Verification items for the finished model (mm, model axes). Face numbers are marked on the shaded views. A direction names the side the tool comes from. Coordinates: 2 decimals unless noted, no trailing zeros. Write each loop counter-clockwise with the first axis right and the second up, starting at its lowest first coordinate (ties: lowest second). Pieces come first, ordered by that corner, then holes. Notation, with made-up numbers: M 77,26.5 L 120,26.5 A21 cw 120,54.5 Z; hole C 52.5,33.25 d6. An arc over 180 degrees is marked long. Answer in a Markdown table with one row per item.
from build123d import *

# Parameters (mm, degrees)
F0_R     = 3
F0_R_2   = 1.5
F1_DEPTH = 2
F0_W     = 43.5258374241
F0_H     = 104
F2_DEPTH = 5
F4_R     = 6.5
F5_DEPTH = 4
F6_R     = 5
F7_R     = 8


# Not quite as in the source:
# - a feature names something its author has since deleted; it is built from what else it names


with BuildPart() as f1:
    # F0 (on Top) → F1 (new body)
    with BuildSketch(Plane.XY):
        Polygon((21, 52), (20, 52), (-20, 52), (-21, 52), (-21, -52), (-20, -52), (20, -52), (21, -52), align=None)
        with Locations((-13, -44)):
            Circle(F0_R, mode=Mode.SUBTRACT)
        with Locations((13, -44)):
            Circle(F0_R, mode=Mode.SUBTRACT)
        with Locations((-13, -8)):
            Circle(F0_R, mode=Mode.SUBTRACT)
        Polygon((-5, -16), (-5, -5), (5, -5), (5, -16), (16, -16), (16, -36), (5, -36), (5, -47), (-5, -47), (-5, -36), (-16, -36), (-16, -16), align=None, mode=Mode.SUBTRACT)
        with Locations((13, -8)):
            Circle(F0_R, mode=Mode.SUBTRACT)
        with Locations((-13, 8)):
            Circle(F0_R, mode=Mode.SUBTRACT)
        with Locations((13, 8)):
            Circle(F0_R, mode=Mode.SUBTRACT)
        with Locations((-13, 44)):
            Circle(F0_R, mode=Mode.SUBTRACT)
        Polygon((-5, 36), (-5, 47), (5, 47), (5, 36), (16, 36), (16, 16), (5, 16), (5, 5), (-5, 5), (-5, 16), (-16, 16), (-16, 36), align=None, mode=Mode.SUBTRACT)
        with Locations((13, 44)):
            Circle(F0_R, mode=Mode.SUBTRACT)
        with Locations((-13, 8)):
            Circle(F0_R)
        with Locations((-13, 8)):
            Circle(F0_R_2, mode=Mode.SUBTRACT)
        with Locations((-13, 44)):
            Circle(F0_R)
        with Locations((-13, 44)):
            Circle(F0_R_2, mode=Mode.SUBTRACT)
    extrude(amount=F1_DEPTH)

    # F0 (on Top) → F2, piece 2 (join)
    with BuildSketch(Plane.XY):
        with Locations((-13, 8)):
            Circle(F0_R)
        with Locations((-13, 8)):
            Circle(F0_R_2, mode=Mode.SUBTRACT)
        with Locations((-13, 44)):
            Circle(F0_R)
        with Locations((-13, 44)):
            Circle(F0_R_2, mode=Mode.SUBTRACT)
        with Locations((13, 44)):
            Circle(F0_R)
        with Locations((13, 44)):
            Circle(F0_R_2, mode=Mode.SUBTRACT)
        with Locations((13, 8)):
            Circle(F0_R)
        with Locations((13, 8)):
            Circle(F0_R_2, mode=Mode.SUBTRACT)
        with Locations((-13, -8)):
            Circle(F0_R)
        with Locations((-13, -8)):
            Circle(F0_R_2, mode=Mode.SUBTRACT)
        with Locations((13, -8)):
            Circle(F0_R)
        with Locations((13, -8)):
            Circle(F0_R_2, mode=Mode.SUBTRACT)
        with Locations((-13, -44)):
            Circle(F0_R)
        with Locations((-13, -44)):
            Circle(F0_R_2, mode=Mode.SUBTRACT)
        with Locations((13, -44)):
            Circle(F0_R)
        with Locations((13, -44)):
            Circle(F0_R_2, mode=Mode.SUBTRACT)
    extrude(amount=F2_DEPTH)


with BuildPart() as f1b:
    # F0 (on Top) → F1, piece 2 (new body)
    with BuildSketch(Plane.XY):
        with Locations((-80.2370812879, 0)):
            Rectangle(F0_W, F0_H)
        with Locations((-69, -44)):
            Circle(F0_R, mode=Mode.SUBTRACT)
        Polygon((-77, -47), (-92, -47), (-92, -5), (-77, -5), (-77, -16), (-63.4741625759, -16), (-63.4741625759, -36), (-77, -36), align=None, mode=Mode.SUBTRACT)
        with Locations((-69, -8)):
            Circle(F0_R, mode=Mode.SUBTRACT)
        with Locations((-69, 8)):
            Circle(F0_R, mode=Mode.SUBTRACT)
        Polygon((-92, 47), (-77, 47), (-77, 36), (-63.4741625759, 36), (-63.4741625759, 16), (-77, 16), (-77, 5), (-92, 5), align=None, mode=Mode.SUBTRACT)
        with Locations((-69, 44)):
            Circle(F0_R, mode=Mode.SUBTRACT)
    extrude(amount=F1_DEPTH)

    # F0 (on Top) → F2 (join)
    with BuildSketch(Plane.XY):
        with Locations((-69, 44)):
            Circle(F0_R)
        with Locations((-69, 44)):
            Circle(F0_R_2, mode=Mode.SUBTRACT)
        with Locations((-69, 8)):
            Circle(F0_R)
        with Locations((-69, 8)):
            Circle(F0_R_2, mode=Mode.SUBTRACT)
        with Locations((-69, -8)):
            Circle(F0_R)
        with Locations((-69, -8)):
            Circle(F0_R_2, mode=Mode.SUBTRACT)
        with Locations((-69, -44)):
            Circle(F0_R)
        with Locations((-69, -44)):
            Circle(F0_R_2, mode=Mode.SUBTRACT)
    extrude(amount=F2_DEPTH)

    # F4 (on face) → F5 (join)
    with BuildSketch(Plane(origin=(-102, 0, 0), x_dir=(0, -1, 0), z_dir=(-1, 0, 0))):
        Polygon((-16, 27.1253478074), (-35.9944990628, 27.1253478074), (-35.9944990628, 0), (-16, 0.4690492824), align=None)
        with Locations((-25.9972495314, 15.1253478074)):
            Circle(F4_R, mode=Mode.SUBTRACT)
        Polygon((16, 0.4690492824), (35.9944990628, 0), (35.9944990628, 27.1253478074), (16, 27.1253478074), align=None)
        with Locations((25.9972495314, 15.1253478074)):
            Circle(F4_R, mode=Mode.SUBTRACT)
    extrude(amount=-F5_DEPTH)

    # F6
    f6_edges = [f1b.edges().sort_by_distance(p)[0] for p in [
        (-98, 25.99725, 2),
        (-98, -25.99725, 2),
    ]]
    fillet(f6_edges, radius=F6_R)

    # F7
    f7_edges = [f1b.edges().sort_by_distance(p)[0] for p in [
        (-100, 35.994499, 27.125348),
        (-100, -16, 27.125348),
        (-100, 16, 27.125348),
        (-100, -35.994499, 27.125348),
    ]]
    fillet(f7_edges, radius=F7_R)


solid = f1b.part
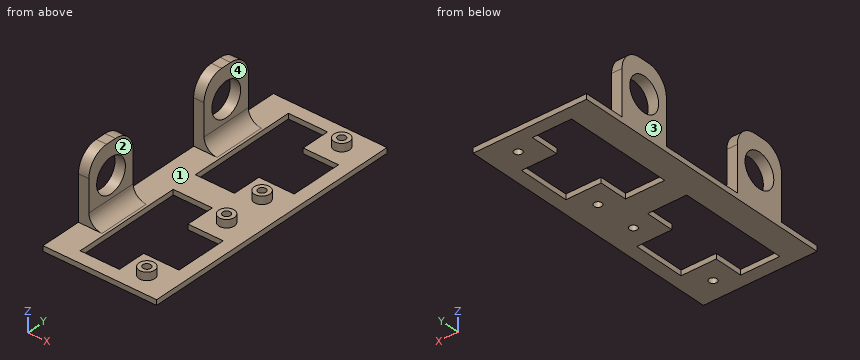
1) Depth check by flat-ended pin: pin 1 (1.8 mm diameter, centred on x = -69, y = -44, fed in from -Z); pin 2 (12 mm diameter, centred on y = 20.5, z = 22, fed in from +X); pin 3 (5 mm diameter, centred on x = -70, y = 8, fed in from +Z); pin 4 (4.5 mm diameter, centred on x = -97, z = 7, fed in from +Y). Enter the tip coordinate at first touch or a pass-through.
Response values:
| item | result |
|---|---|
| pin 1 | passes through |
| pin 2 | stops at x = -98 |
| pin 3 | stops at z = 5 |
| pin 4 | stops at y = 35.99 |
2) Release check for a two-part mould opening along Y. For the marked faces 1 and 2 record: +Y half, -Y half, draft (parallel to the pull), parting line (faces both ways), or undercut.
Response values:
| item | result |
|---|---|
| face 1 | undercut |
| face 2 | draft |
3) Sectioned sample at D-D (x = -69). Give the number of separate pieces and of enclosed holes in the cut face, then the cut area to 3 significant figures.
Response values:
| item | result |
|---|---|
| separate pieces | 7 |
| enclosed holes | 0 |
| area | 140 mm² |
4) Thickness scan on L1, parallel to Y at x = -100, z = 9.5; L2, parallel to Z at x = -71, y = -11; L3, parallel to X at y = 32.5, z = 19. Record the ranges inside material, lowest first. Write a range as [from, to].
Response values:
| item | result |
|---|---|
| L1 | y = [-35.99, -29.25], [-22.74, -16], [16, 22.74], [29.25, 35.99] |
| L2 | z = [0, 2] |
| L3 | x = [-102, -98] |
5) Sectioned sample at B-B (x = -85). Record the cut outline in (y, z), then the cut area to 3 significant figures.
Response values:
| item | result |
|---|---|
| outline | M -52,0 L -47,0 L -47,2 L -52,2 Z; M -5,0 L 5,0 L 5,2 L -5,2 Z; M 47,0 L 52,0 L 52,2 L 47,2 Z |
| area | 40.0 mm² |
6) Sectioned sample at A-A (y = 44). Record the cut outline in (x, z).
Response values:
| item | result |
|---|---|
| outline | M -102,0 L -92,0 L -92,2 L -102,2 Z; M -77,0 L -70.5,0 L -70.5,5 L -72,5 L -72,2 L -77,2 Z; M -67.5,0 L -58.47,0 L -58.47,2 L -66,2 L -66,5 L -67.5,5 Z |
7) Sectioned sample at C-C (z = 17.5). Record the cut outline in (x, y), then the cut area to 3 significant figures.
Response values:
| item | result |
|---|---|
| outline | M -102,-35.99 L -98,-35.99 L -98,-32.05 L -102,-32.05 Z; M -102,-19.95 L -98,-19.95 L -98,-16 L -102,-16 Z; M -102,16 L -98,16 L -98,19.95 L -102,19.95 Z; M -102,32.05 L -98,32.05 L -98,35.99 L -102,35.99 Z |
| area | 63.1 mm² |
8) Tool access check on the marked faces 3 and 4. Record the directions out of +Z, -Z, +X, -X, +Y, -Y that give a thin tool (end or side, any length) a straight path to the whole face; none if there is none.
Response values:
| item | result |
|---|---|
| face 3 | +Z, -Z, -X, +Y, -Y |
| face 4 | +Z, +X, +Y, -Y |
